```python
from build123d import *

# Parameters (mm, degrees)
EXTRUDE_2_DEPTH     = 5
SKETCH_3_R          = 1.5
CUT_EXTRUDE_1_DEPTH = 10


with BuildPart() as part:
    # Эскиз1 → Бобышка-Вытянуть2 (new, symmetric)
    with BuildSketch(Plane.XY):
        with BuildLine():
            Line((-15, -55), (-15, -65))
            Line((-15, -65), (-25, -65))
            Line((-25, -65), (-25, -55))
            Line((-25, -55), (-35, -55))
            Line((-35, -55), (-35, -65))
            Line((-35, -65), (-45, -65))
            Line((-45, -65), (-45, -55))
            Line((-45, -55), (-45, 45))
            ThreePointArc((-45, 45), (-42.071067812, 52.071067812), (-35, 55))
            Line((-35, 55), (35, 55))
            ThreePointArc((35, 55), (42.071067812, 52.071067812), (45, 45))
            Line((45, 45), (45, -55))
            Line((45, -55), (45, -65))
            Line((45, -65), (35, -65))
            Line((35, -65), (35, -55))
            Line((35, -55), (25, -55))
            Line((25, -55), (25, -65))
            Line((25, -65), (15, -65))
            Line((15, -65), (15, -55))
            Line((15, -55), (5, -55))
            Line((5, -55), (5, -65))
            Line((5, -65), (-5, -65))
            Line((-5, -65), (-5, -55))
            Line((-5, -55), (-15, -55))
        make_face()
    extrude(amount=EXTRUDE_2_DEPTH, both=True)

    # Эскиз3 → Вырез-Вытянуть1 (cut)
    with BuildSketch(Plane.XY.offset(5)):
        with Locations((-34, 44)):
            Circle(SKETCH_3_R)
        with Locations((34, 44)):
            Circle(SKETCH_3_R)
        with Locations((34, -38)):
            Circle(SKETCH_3_R)
        with Locations((-34, -38)):
            Circle(SKETCH_3_R)
    extrude(amount=-CUT_EXTRUDE_1_DEPTH, mode=Mode.SUBTRACT)


solid = part.part
```
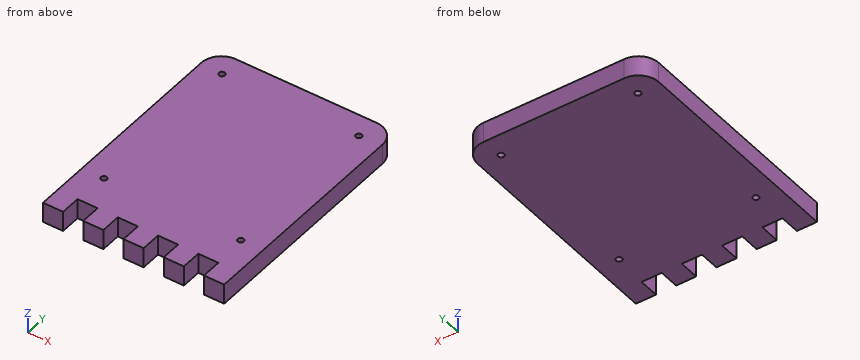
Here's how the part is built. I have some questions about the finished solid (model axes, mm). Round coordinates to 2 decimals unless told otherwise and drop trailing zeros. Write each loop counter-clockwise with the first axis right and the second up, starting at its lowest first coordinate (ties: lowest second). Pieces come first, ordered by that corner, then holes. Notation, with made-up numbers: M 29.25,56.5 L 64.25,56.5 A24 ccw 64.25,81.5 Z; hole C 34,36 d6. An arc over 180 degrees is marked long. Answer as CSV lines item,"result". Start each with the question number.
1. Suppose I cut it at C-C on x = 27. Write out the boundary of the cut face in (y, z), then the cut area to 3 significant figures.
2. I'm going to push flat-ended pins straight in: pin 1 Ø5 at (x, z) = (-28, 0) entering from -Y; pin 2 Ø2.5 at (x, y) = (34, 44) entering from +Z. Where does each tip first touch, or does it pass through?
3. Suppose I cut it at B-B on z = -1. Write out the boundary of the cut face in (x, y), then the cut area to 3 significant figures.
4. I need wall thicknesses on probe 1 along Y at (x, z) = (-34, -2.75); probe 2 along Y at (x, z) = (13, 1.5). Which ranges of each line are inside material? Lowest first, please.
5. Suppose I cut it at A-A on y = -38. Write out the boundary of the cut face in (x, z).
Check result:
1,outline,"M -55,-5 L 55,-5 L 55,5 L -55,5 Z"
1,area,"1,100 mm2"
2,pin 1,"stops at y = -55"
2,pin 2,"passes through"
3,outline,"M -45,-65 L -35,-65 L -35,-55 L -25,-55 L -25,-65 L -15,-65 L -15,-55 L -5,-55 L -5,-65 L 5,-65 L 5,-55 L 15,-55 L 15,-65 L 25,-65 L 25,-55 L 35,-55 L 35,-65 L 45,-65 L 45,45 A10 ccw 35,55 L -35,55 A10 ccw -45,45 Z; hole C -34,-38 d3; hole C -34,44 d3; hole C 34,-38 d3; hole C 34,44 d3"
3,area,"10,300 mm2"
4,probe 1,"y = -55 to -39.5, -36.5 to 42.5, 45.5 to 55"
4,probe 2,"y = -55 to 55"
5,outline,"M -45,-5 L -35.5,-5 L -35.5,5 L -45,5 Z; M -32.5,-5 L 32.5,-5 L 32.5,5 L -32.5,5 Z; M 35.5,-5 L 45,-5 L 45,5 L 35.5,5 Z"
